The model under review builds one solid part; all positions refer to its coordinate system, in mm. A direction names the side the tool comes from. Coordinates: 2 decimals unless noted, no trailing zeros. Order: outer loops, then holes, each group sorted by start corner. A loop starts at its lowest first (then second) coordinate and runs counter-clockwise, first axis right, second up. Notation, with made-up numbers: (-27, 15.5) -> (-6, 15.5) arc R23 ccw to (-6, 34.5) -> close; hole circle Ø7 at (75, -32). An arc over 180 degrees is marked (long way). Use one line per item in the form item = value. Start each with the question number.
(1) Wall thickness on line 1 along X through (y, z) = (0.65, -32) (3 decimals); line 2 along X through (y, z) = (1.85, -30.5) (3 decimals); line 3 along Z through (x, y) = (17, 0.6) (3 decimals): over which ranges is each line inside the solid? List them lowest first.
(2) Take a section at B-B (x = -18). State the section outline as (y, z) points (3 decimals).
(3) For faces 5 (the flat face through (41.825, 2, -28)), 6 (the flat face through (-41.825, 2, 28)), 7 (the flat face through (-20, 2, -33)), 8 (the flat face through (-43, 2, -20.25)), 9 (the flat face through (20, 2, 33)), list the 3-axis set-ups (+Z, -Z, +X, -X, +Y, -Y) from which the entire face can be reached by the end or side of a thin tool; tool diameter is ignored.
(4) Take a section at A-A (y = 0.75). State the section outline as (x, z) points (3 decimals), then the cut area to 3 significant figures.
(5) Insertion check: pin 1 Ø1.6 at (x, y) = (-7.5, 2) entering from +Z (3 decimals); pin 2 Ø1.6 at (x, y) = (43.5, 1) entering from -Z; pin 3 Ø1 at (x, y) = (-13.5, 0.5) entering from -Z (3 decimals); pin 4 Ø1 at (x, z) = (-1.5, -24) entering from -Y. Each pin has a flat end and moves straight along its axis. Give the tip position at first contact, or say it passes through.
(6) Mouldability with a two-part tool opening along X and no side actions: class faces 1 (the flat face through (41.825, 2, 28)), 2 (the flat face through (31, 2, -35)), 3 (the flat face through (0, 2, 31.825)), 4 (the flat face through (-45, 2, 0)) as +X half, -X half, draft (parallel to the pull), parting line (faces both ways), or undercut.
(7) Take a section at C-C (z = -28). State the section outline as (x, y) points (3 decimals).
```python
from build123d import *

# Parameters (mm, degrees)
SKETCH1_W           = 21.825
SKETCH1_H           = 3.175
SKETCH1_W_2         = 3.175
SKETCH1_H_2         = 40.5
BOSS_EXTRUDE1_DEPTH = 3.175


with BuildPart() as part:
    # Sketch1 → Boss-Extrude1 (new body)
    with BuildSketch(Plane(origin=(0, 0, 0), x_dir=(1, 0, 0), z_dir=(0, 1, 0))):
        Polygon((-20, 31.825), (-41.825, 31.825), (-41.825, 20.25), (-41.825, -20.25), (-41.825, -31.825), (-20, -31.825), (20, -31.825), (41.825, -31.825), (41.825, -20.25), (41.825, 20.25), (41.825, 31.825), (20, 31.825), align=None)
        with Locations((-30.9125, -33.4125)):
            Rectangle(SKETCH1_W, SKETCH1_H)
        with Locations((30.9125, -33.4125)):
            Rectangle(SKETCH1_W, SKETCH1_H)
        with Locations((43.4125, 0)):
            Rectangle(SKETCH1_W_2, SKETCH1_H_2)
        with Locations((30.9125, 33.4125)):
            Rectangle(SKETCH1_W, SKETCH1_H)
        with Locations((-30.9125, 33.4125)):
            Rectangle(SKETCH1_W, SKETCH1_H)
        with Locations((-43.4125, 0)):
            Rectangle(SKETCH1_W_2, SKETCH1_H_2)
    extrude(amount=BOSS_EXTRUDE1_DEPTH)


solid = part.part
```
Findings:
q1.line_1 = -41.825 to -20, 20 to 41.825
q1.line_2 = -41.825 to 41.825
q1.line_3 = -31.825 to 31.825
q2.outline = (0, -31.825) -> (3.175, -31.825) -> (3.175, 31.825) -> (0, 31.825) -> close
q3.face_5 = -Z, +X, +Y, -Y
q3.face_6 = +Z, -X, +Y, -Y
q3.face_7 = -Z, +Y, -Y
q3.face_8 = -Z, -X, +Y, -Y
q3.face_9 = +Z, +Y, -Y
q4.outline = (-45, -20.25) -> (-41.825, -20.25) -> (-41.825, -35) -> (-20, -35) -> (-20, -31.825) -> (20, -31.825) -> (20, -35) -> (41.825, -35) -> (41.825, -20.25) -> (45, -20.25) -> (45, 20.25) -> (41.825, 20.25) -> (41.825, 35) -> (20, 35) -> (20, 31.825) -> (-20, 31.825) -> (-20, 35) -> (-41.825, 35) -> (-41.825, 20.25) -> (-45, 20.25) -> close
q4.area = 5,860 mm²
q5.pin_1 = 31.825
q5.pin_2 = -20.25
q5.pin_3 = -31.825
q5.pin_4 = 0
q6.face_1 = +X half
q6.face_2 = draft
q6.face_3 = undercut
q6.face_4 = -X half
q7.outline = (-41.825, 0) -> (41.825, 0) -> (41.825, 3.175) -> (-41.825, 3.175) -> close
